from build123d import *

# Parameters (mm, degrees)
SKETCH_1_R      = 5.025
EXTRUDE_1_DEPTH = 8


with BuildPart() as part:
    # 草图1 → 凸台-拉伸1 (new body)
    with BuildSketch(Plane.XY):
        with BuildLine():
            Line((-15, 0), (-15, -200))
            ThreePointArc((-15, -200), (0, -215), (15, -200))
            Line((15, -200), (15, 0))
            ThreePointArc((15, 0), (0, 15), (-15, 0))
        make_face()
        Circle(SKETCH_1_R, mode=Mode.SUBTRACT)
        with Locations((0, -200)):
            Circle(SKETCH_1_R, mode=Mode.SUBTRACT)
        with BuildLine():
            Line((-9, -16.970562748), (-9, -57.5))
            ThreePointArc((-9, -57.5), (0, -66.5), (9, -57.5))
            Line((9, -57.5), (9, -16.970562748))
            ThreePointArc((9, -16.970562748), (7.732050808, -14.521073006), (5, -14.142135624))
            ThreePointArc((5, -14.142135624), (0, -15), (-5, -14.142135624))
            ThreePointArc((-5, -14.142135624), (-7.732050808, -14.521073006), (-9, -16.970562748))
        make_face(mode=Mode.SUBTRACT)
        with BuildLine():
            Line((9, -82.5), (9, -117.5))
            ThreePointArc((9, -117.5), (0, -126.5), (-9, -117.5))
            Line((-9, -117.5), (-9, -82.5))
            ThreePointArc((-9, -82.5), (0, -73.5), (9, -82.5))
        make_face(mode=Mode.SUBTRACT)
        with BuildLine():
            Line((-9, -183.029437252), (-9, -142.5))
            ThreePointArc((-9, -142.5), (0, -133.5), (9, -142.5))
            Line((9, -142.5), (9, -183.029437252))
            ThreePointArc((9, -183.029437252), (7.732050808, -185.478926994), (5, -185.857864376))
            ThreePointArc((5, -185.857864376), (0, -185), (-5, -185.857864376))
            ThreePointArc((-5, -185.857864376), (-7.732050808, -185.478926994), (-9, -183.029437252))
        make_face(mode=Mode.SUBTRACT)
    extrude(amount=EXTRUDE_1_DEPTH)


solid = part.part
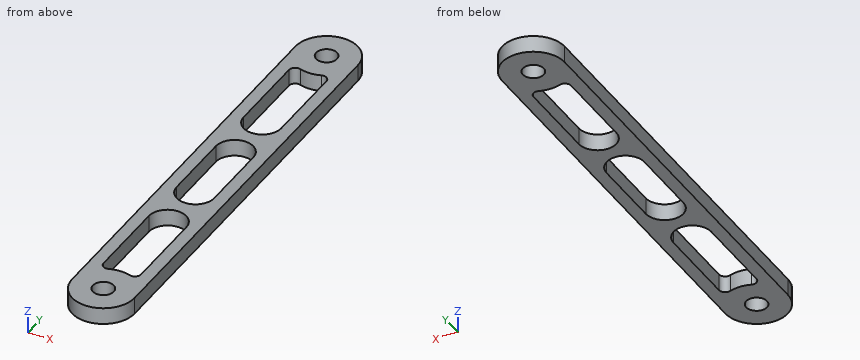
The model under review builds one solid part; all positions refer to its coordinate system, in mm. Coordinates: 2 decimals unless noted, no trailing zeros. Order: outer loops, then holes, each group sorted by start corner. A loop starts at its lowest first (then second) coordinate and runs counter-clockwise, first axis right, second up. Notation, with made-up numbers: (0.25, 6.5) -> (6.25, 6.5) arc R17 ccw to (6.25, 34.5) -> close; hole circle Ø7 at (24.25, 21). An arc over 180 degrees is marked (long way). Answer in a Markdown table with one row per item.
(1) Insertion check: pin 1 (2 mm diameter, centred on x = 11.5, z = 4, fed in from +Y); pin 2 (3 mm diameter, centred on x = -5, z = 5, fed in from +Y); pin 3 (1 mm diameter, centred on x = 9, z = 3.5, fed in from +Y). Each pin has a flat end and moves straight along its axis. Give the tip position at first contact, or say it passes through.
Answers:
| item | result |
|---|---|
| pin 1 | y = 10.71 |
| pin 2 | y = 14.59 |
| pin 3 | y = 12.36 |
(2) Consider section B-B (z = 4.5). Write out the cut boundary in (x, y) (3 decimals), plus the area to 3 significant figures.
Answers:
| item | result |
|---|---|
| outline | (-15, -200) arc R15 ccw to (15, -200) -> (15, 0) arc R15 ccw to (-15, 0) -> close; hole (-9, -183.029) arc R3 ccw to (-5, -185.858) arc R15 cw to (5, -185.858) arc R3 ccw to (9, -183.029) -> (9, -142.5) arc R9 ccw to (-9, -142.5) -> close; hole (-9, -117.5) arc R9 ccw to (9, -117.5) -> (9, -82.5) arc R9 ccw to (-9, -82.5) -> close; hole (-9, -57.5) arc R9 ccw to (9, -57.5) -> (9, -16.971) arc R3 ccw to (5, -14.142) arc R15 cw to (-5, -14.142) arc R3 ccw to (-9, -16.971) -> close; hole circle Ø10.05 at (0, -200); hole circle Ø10.05 at (0, 0) |
| area | 3,870 mm² |
(3) Wall thickness on line 1 along Y through (x, z) = (0, 2) (3 decimals); line 2 along Y through (x, z) = (-2.5, 4); line 3 along Y through (x, z) = (5.5, 4): over which ranges is each line inside the solid? List them lowest first.
Answers:
| item | result |
|---|---|
| line 1 | -215 to -205.025, -194.975 to -185, -133.5 to -126.5, -73.5 to -66.5, -15 to -5.025, 5.025 to 15 |
| line 2 | -214.79 to -204.36, -195.64 to -185.21, -133.85 to -126.15, -73.85 to -66.15, -14.79 to -4.36, 4.36 to 14.79 |
| line 3 | -213.96 to -185.99, -135.38 to -124.62, -75.38 to -64.62, -14.01 to 13.96 |
(4) Consider section C-C (y = -79). Write out the cut boundary in (x, z), plus the area to 3 significant figures.
Answers:
| item | result |
|---|---|
| outline | (-15, 0) -> (-8.29, 0) -> (-8.29, 8) -> (-15, 8) -> close; (8.29, 0) -> (15, 0) -> (15, 8) -> (8.29, 8) -> close |
| area | 107 mm² |
(5) Consider section A-A (x = 0). Write out the cut boundary in (y, z) (3 decimals).
Answers:
| item | result |
|---|---|
| outline | (-215, 0) -> (-205.025, 0) -> (-205.025, 8) -> (-215, 8) -> close; (-194.975, 0) -> (-185, 0) -> (-185, 8) -> (-194.975, 8) -> close; (-133.5, 0) -> (-126.5, 0) -> (-126.5, 8) -> (-133.5, 8) -> close; (-73.5, 0) -> (-66.5, 0) -> (-66.5, 8) -> (-73.5, 8) -> close; (-15, 0) -> (-5.025, 0) -> (-5.025, 8) -> (-15, 8) -> close; (5.025, 0) -> (15, 0) -> (15, 8) -> (5.025, 8) -> close |
